Source: CAD feature listing. Evaluate the final solid. Frame: model axes, mm. Face numbers are marked on the shaded views. Round coordinates to 2 decimals unless told otherwise and drop trailing zeros. Write each loop counter-clockwise with the first axis right and the second up, starting at its lowest first coordinate (ties: lowest second). Pieces come first, ordered by that corner, then holes.
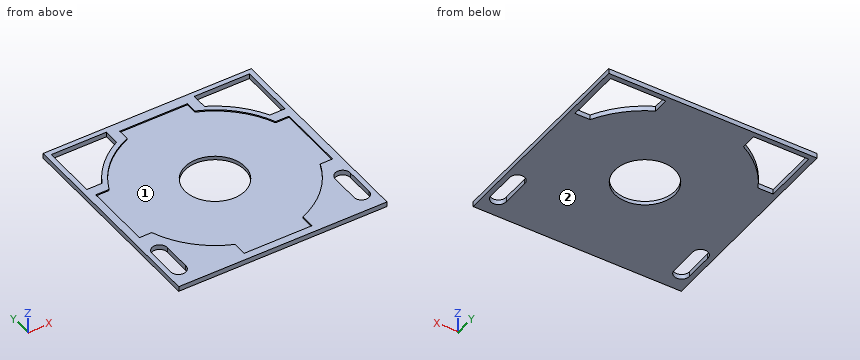
from build123d import *

# Parameters (mm, degrees)
F0_W      = 269.875
F0_H      = 273.05
F1_DEPTH  = 6.35
F3_DEPTH  = 6.35
F4_R      = 38.1
F5_DEPTH  = 6.35
F7_DEPTH  = 1.5875
F8_W      = 3.175
F8_H      = 273.05
F9_DEPTH  = 6.35
F10_W     = 263.525
F10_H     = 3.175
F11_DEPTH = 6.35
F12_W     = 263.525
F12_H     = 3.175
F13_DEPTH = 6.35


with BuildPart() as f1:
    # F0 (on Top) → F1 (new body)
    with BuildSketch(Plane.XY):
        Rectangle(F0_W, F0_H)
    extrude(amount=F1_DEPTH)

    # F2 (on face) → F3 (cut, through all)
    with BuildSketch(Plane.XY.offset(6.35)):
        with BuildLine():
            Line((-55.5625, 127), (-125.4125, 127))
            Line((-125.4125, 127), (-125.4125, 57.15))
            Line((-125.4125, 57.15), (-106.251468, 57.15))
            ThreePointArc((-106.251468, 57.15), (-84.672021, 85.939978), (-55.5625, 107.0864))
            Line((-55.5625, 107.0864), (-55.5625, 127))
        make_face()
        with BuildLine():
            Line((55.5625, 127), (55.5625, 107.0864))
            ThreePointArc((55.5625, 107.0864), (84.672021, 85.939978), (106.251468, 57.15))
            Line((106.251468, 57.15), (125.4125, 57.15))
            Line((125.4125, 57.15), (125.4125, 127))
            Line((125.4125, 127), (55.5625, 127))
        make_face()
        with BuildLine():
            ThreePointArc((-106.3625, -71.485033), (-115.8875, -61.4553), (-125.4125, -71.485033))
            Line((-125.4125, -71.485033), (-125.4125, -107.445267))
            ThreePointArc((-125.4125, -107.445267), (-115.8875, -117.475), (-106.3625, -107.445267))
            Line((-106.3625, -107.445267), (-106.3625, -71.485033))
        make_face()
        with BuildLine():
            ThreePointArc((125.4125, -71.483554), (115.8875, -61.455376), (106.3625, -71.483554))
            Line((106.3625, -71.483554), (106.3625, -107.445267))
            ThreePointArc((106.3625, -107.445267), (115.8875, -117.475), (125.4125, -107.445267))
            Line((125.4125, -107.445267), (125.4125, -71.483554))
        make_face()
    extrude(amount=-F3_DEPTH, mode=Mode.SUBTRACT)

    # F4 (on face) → F5 (cut, through all)
    with BuildSketch(Plane.XY.offset(6.35)):
        Circle(F4_R)
    extrude(amount=-F5_DEPTH, mode=Mode.SUBTRACT)

    # F6 (on face) → F7 (cut)
    with BuildSketch(Plane.XY.offset(6.35)):
        with BuildLine():
            ThreePointArc((106.587356, -41.275), (112.355295, -20.994705), (114.3, 0))
            ThreePointArc((114.3, 0), (112.028131, 22.675711), (105.302837, 44.45))
            Line((105.302837, 44.45), (42.8625, 44.45))
            Line((42.8625, 44.45), (42.8625, 105.958936))
            ThreePointArc((42.8625, 105.958936), (0, 114.3), (-42.8625, 105.958936))
            Line((-42.8625, 105.958936), (-42.8625, 44.45))
            Line((-42.8625, 44.45), (-105.302837, 44.45))
            ThreePointArc((-105.302837, 44.45), (-114.287171, 1.712499), (-106.587356, -41.275))
            Line((-106.587356, -41.275), (-42.8625, -41.275))
            Line((-42.8625, -41.275), (-42.8625, -105.958936))
            ThreePointArc((-42.8625, -105.958936), (0, -114.3), (42.8625, -105.958936))
            Line((42.8625, -105.958936), (42.8625, -41.275))
            Line((42.8625, -41.275), (106.587356, -41.275))
        make_face()
        with BuildLine():
            ThreePointArc((105.302837, 44.45), (112.028131, 22.675711), (114.3, 0))
            ThreePointArc((114.3, 0), (112.355295, -20.994705), (106.587356, -41.275))
            Line((106.587356, -41.275), (122.2375, -41.275))
            Line((122.2375, -41.275), (122.2375, 44.45))
            Line((122.2375, 44.45), (105.302837, 44.45))
        make_face()
        with BuildLine():
            Line((42.8625, 44.45), (105.302837, 44.45))
            ThreePointArc((105.302837, 44.45), (80.212711, 81.427335), (42.8625, 105.958936))
            Line((42.8625, 105.958936), (42.8625, 44.45))
        make_face()
        with BuildLine():
            ThreePointArc((42.8625, -105.958936), (81.423693, -80.216409), (106.587356, -41.275))
            Line((106.587356, -41.275), (42.8625, -41.275))
            Line((42.8625, -41.275), (42.8625, -105.958936))
        make_face()
        with BuildLine():
            ThreePointArc((-42.8625, 105.958936), (0, 114.3), (42.8625, 105.958936))
            Line((42.8625, 105.958936), (42.8625, 120.65))
            Line((42.8625, 120.65), (-42.8625, 120.65))
            Line((-42.8625, 120.65), (-42.8625, 105.958936))
        make_face()
        with BuildLine():
            Line((42.8625, -123.825), (42.8625, -105.958936))
            ThreePointArc((42.8625, -105.958936), (0, -114.3), (-42.8625, -105.958936))
            Line((-42.8625, -105.958936), (-42.8625, -123.825))
            Line((-42.8625, -123.825), (42.8625, -123.825))
        make_face()
        with BuildLine():
            Line((-42.8625, 44.45), (-42.8625, 105.958936))
            ThreePointArc((-42.8625, 105.958936), (-80.212711, 81.427335), (-105.302837, 44.45))
            Line((-105.302837, 44.45), (-42.8625, 44.45))
        make_face()
        with BuildLine():
            ThreePointArc((-106.587356, -41.275), (-81.423693, -80.216409), (-42.8625, -105.958936))
            Line((-42.8625, -105.958936), (-42.8625, -41.275))
            Line((-42.8625, -41.275), (-106.587356, -41.275))
        make_face()
        with BuildLine():
            ThreePointArc((-106.587356, -41.275), (-114.287171, 1.712499), (-105.302837, 44.45))
            Line((-105.302837, 44.45), (-122.2375, 44.45))
            Line((-122.2375, 44.45), (-122.2375, -41.275))
            Line((-122.2375, -41.275), (-106.587356, -41.275))
        make_face()
    extrude(amount=-F7_DEPTH, mode=Mode.SUBTRACT)

    # F8 (on face) → F9 (cut, through all)
    with BuildSketch(Plane.XY.offset(6.35)):
        with Locations((-133.35, 0)):
            Rectangle(F8_W, F8_H)
        with Locations((133.35, 0)):
            Rectangle(F8_W, F8_H)
    extrude(amount=-F9_DEPTH, mode=Mode.SUBTRACT)

    # F10 (on face) → F11 (cut, through all)
    with BuildSketch(Plane.XY.offset(6.35)):
        with Locations((0, 134.9375)):
            Rectangle(F10_W, F10_H)
    extrude(amount=-F11_DEPTH, mode=Mode.SUBTRACT)

    # F12 (on face) → F13 (cut, through all)
    with BuildSketch(Plane.XY.offset(6.35)):
        with Locations((0, -134.9375)):
            Rectangle(F12_W, F12_H)
    extrude(amount=-F13_DEPTH, mode=Mode.SUBTRACT)


solid = f1.part
1) Section query B-B on z = 2.5. Return the cut outline in (x, y), then the cut area to 3 significant figures.
Taken from the geometry:
outline: (-131.76, -133.35) - (131.76, -133.35) - (131.76, 133.35) - (-131.76, 133.35) - close; hole (-125.41, -107.45) arc R9.54 ccw (long way) to (-106.36, -107.45) - (-106.36, -71.49) arc R9.54 ccw (long way) to (-125.41, -71.49) - close; hole (-125.41, 57.15) - (-106.25, 57.15) arc R120.65 cw to (-55.56, 107.09) - (-55.56, 127) - (-125.41, 127) - close; hole circle Ø76.2 at (0, 0); hole (55.56, 107.09) arc R120.65 cw to (106.25, 57.15) - (125.41, 57.15) - (125.41, 127) - (55.56, 127) - close; hole (106.36, -107.45) arc R9.54 ccw (long way) to (125.41, -107.45) - (125.41, -71.48) arc R9.54 ccw (long way) to (106.36, -71.48) - close
area: 57,000 mm2
2) Contact query for a flat-ended pin moving along its axis: P1, Ø12, axis at x = 54, y = -91, coming from the +Z side. Output: stop coordinate, or through.
Taken from the geometry:
P1: stops at z = 4.76
3) Pull-direction query (Y, two-part tool) for the marked faces 1 and 2; classes: released by +Y, released by -Y, zero draft, split by the parting line, or undercut.
Taken from the geometry:
face 1: undercut
face 2: zero draft
4) Material intervals for line 1 (X direction, y = 107.5, z = 2); line 2 (X direction, y = -76, z = 2.75); line 3 (Y direction, x = -115, z = 3.5), sorted ascending.
Taken from the geometry:
line 1: x = -131.76 to -125.41, -55.56 to 55.56, 125.41 to 131.76
line 2: x = -131.76 to -125.41, -106.36 to 106.36, 125.41 to 131.76
line 3: y = -133.35 to -117.43, -61.5 to 57.15, 127 to 133.35
5) Section query D-D on y = 79. Return the cut outline in (x, z), then the cut area to 3 significant figures.
Taken from the geometry:
outline: (-131.76, 0) - (-125.41, 0) - (-125.41, 6.35) - (-131.76, 6.35) - close; (-91.18, 0) - (91.18, 0) - (91.18, 6.35) - (82.6, 6.35) - (82.6, 4.76) - (-82.6, 4.76) - (-82.6, 6.35) - (-91.18, 6.35) - close; (125.41, 0) - (131.76, 0) - (131.76, 6.35) - (125.41, 6.35) - close
area: 976 mm2
6) Section query C-C on y = 0. Return the cut outline in (x, z), then the cut area to 3 significant figures.
Taken from the geometry:
outline: (-131.76, 0) - (-38.1, 0) - (-38.1, 4.76) - (-122.24, 4.76) - (-122.24, 6.35) - (-131.76, 6.35) - close; (38.1, 0) - (131.76, 0) - (131.76, 6.35) - (122.24, 6.35) - (122.24, 4.76) - (38.1, 4.76) - close
area: 922 mm2
